Could you check a few things on this model? Use its own coordinates, in mm. A direction names the side the tool comes from. Coordinates: 2 decimals unless noted, no trailing zeros. Order: outer loops, then holes, each group sorted by start corner. A loop starts at its lowest first (then second) coordinate and runs counter-clockwise, first axis right, second up. Notation, with made-up numbers: (75, 20) - (124, 20) arc R20 cw to (124, 59) - close; hole circle Ø4 at (33, -23). An arc over 180 degrees is marked (long way). Answer as a JSON object with one key per item and string values. Group by question number.
(1) Please list where these lines run through material, in increasing order: probe 1 along Y at (x, z) = (0, -2.1); probe 2 along Y at (x, z) = (0, 1.25); probe 3 along X at (y, z) = (0, 2.35).
(2) Will these pins go through, and if not, where does the flat tip stop? P1, Ø1, axis at y = -16.5, z = 1, coming from the -X side; P2, Ø19.5, axis at x = -3, y = 1, coming from the +Z side; P3, Ø2, axis at x = -44.5, z = -1, coming from the -Y side.
(3) Imagine slicing it at A-A, the plane x = 0. Write out the boundary of the cut face in (y, z).
(4) Imagine slicing it at B-B, the plane y = 26. Write out the boundary of the cut face in (x, z), and give its area (3 significant figures).
(5) Imagine slicing it at C-C, the plane z = 1.75. Write out the boundary of the cut face in (x, y), and give its area (3 significant figures).
(6) We'd pull the mould along Y, two halves only. Please class faces 3 (the flat face through (-14, 14, 3.25)), 4 (the cylindrical face through (-1.38, 6.2, -1.48)), 5 (the cylindrical face through (26.76, 51.46, -1.52)): pulls with the +Y half, pulls with the -Y half, needs draft (parallel to the pull), parting line crosses it, or undercut.
(7) Imagine slicing it at D-D, the plane y = -13. Write out the boundary of the cut face in (x, z) (3 decimals).
(8) Which directions (+Z, -Z, +X, -X, +Y, -Y) give clear straight access to the entire face, cutting with the end or side of a thin tool? Please do faces 1 (the cylindrical face through (-22.159, -10.273, 0.081)), 2 (the cylindrical face through (-7.13, 32.12, 1.6)).
from build123d import *

# Parameters (mm, degrees)
M5_CLEARANCE_HOLE1_D = 5.5


with BuildPart() as part:
    # Sketch4 → Revolve1 (revolve)
    with BuildSketch(Plane(origin=(0, 0, 0), x_dir=(1, 0, 0), z_dir=(0, 1, 0))):
        Polygon((6.35, 0), (19.3, 0), (19.3, -3.25), (32.9, -3.25), (32.9, 0), (58, 0), (58, 3), (6.35, 3), align=None)
    revolve(axis=Axis((0, 0, 0), (0, 0, -1)))

    # M5 Clearance Hole1 (through all)
    with Locations(Plane.XY.offset(3.25)):
        with Locations((0, 26), (-22.516660498, -13), (22.516660498, -13)):
            Hole(M5_CLEARANCE_HOLE1_D / 2)


solid = part.part
Result set:
{
 "1": {"probe 1": "y = -58 to -6.35, 6.35 to 23.25, 28.75 to 58", "probe 2": "y = -32.9 to -19.3, 19.3 to 23.25, 28.75 to 32.9", "probe 3": "x = -32.9 to -19.3, 19.3 to 32.9"},
 "2": {"P1": "stops at x = -28.75", "P2": "stops at z = 0", "P3": "stops at y = -38.36"},
 "3": {"outline": "(-58, -3) - (-6.35, -3) - (-6.35, 0) - (-19.3, 0) - (-19.3, 3.25) - (-32.9, 3.25) - (-32.9, 0) - (-58, 0) - close; (6.35, -3) - (23.25, -3) - (23.25, 3.25) - (19.3, 3.25) - (19.3, 0) - (6.35, 0) - close; (28.75, -3) - (58, -3) - (58, 0) - (32.9, 0) - (32.9, 3.25) - (28.75, 3.25) - close"},
 "4": {"outline": "(-51.85, -3) - (-2.75, -3) - (-2.75, 3.25) - (-20.16, 3.25) - (-20.16, 0) - (-51.85, 0) - close; (2.75, -3) - (51.85, -3) - (51.85, 0) - (20.16, 0) - (20.16, 3.25) - (2.75, 3.25) - close", "area": "408 mm^2"},
 "5": {"outline": "circle Ø65.8 at (0, 0); hole circle Ø5.5 at (-22.52, -13); hole circle Ø38.6 at (0, 0); hole circle Ø5.5 at (0, 26); hole circle Ø5.5 at (22.52, -13)", "area": "2,160 mm^2"},
 "6": {"face 3": "needs draft", "face 4": "undercut", "face 5": "parting line crosses it"},
 "7": {"outline": "(-56.524, -3) - (-25.267, -3) - (-25.267, 3.25) - (-30.223, 3.25) - (-30.223, 0) - (-56.524, 0) - close; (-19.767, -3) - (19.767, -3) - (19.767, 3.25) - (14.265, 3.25) - (14.265, 0) - (-14.265, 0) - (-14.265, 3.25) - (-19.767, 3.25) - close; (25.267, -3) - (56.524, -3) - (56.524, 0) - (30.223, 0) - (30.223, 3.25) - (25.267, 3.25) - close"},
 "8": {"face 1": "+Z, -Z", "face 2": "+Z"}
}
